from build123d import *

# Parameters (mm, degrees)
SKETCH1_R            = 36.5
BOSS_EXTRUDE1_DEPTH  = 5
SKETCH2_W            = 22
SKETCH2_H            = 14
CUT_EXTRUDE1_DEPTH   = 2.5
SKETCH6_W            = 14
SKETCH6_H            = 1.2
BOSS_EXTRUDE2_DEPTH  = 2.1
SKETCH7_W            = 14
SKETCH7_H            = 1.2
BOSS_EXTRUDE3_DEPTH  = 2.1
SKETCH8_W            = 14
SKETCH8_H            = 1.2
BOSS_EXTRUDE4_DEPTH  = 2.1
SKETCH10_W           = 14
SKETCH10_H           = 1.2
BOSS_EXTRUDE10_DEPTH = 2.1
SKETCH21_W           = 14
SKETCH21_H           = 1.2
BOSS_EXTRUDE11_DEPTH = 2.1
SKETCH13_W           = 14
SKETCH13_H           = 1.2
BOSS_EXTRUDE7_DEPTH  = 2.1
SKETCH14_W           = 14
SKETCH14_H           = 1.2
BOSS_EXTRUDE8_DEPTH  = 2.1
SKETCH18_W           = 14
SKETCH18_H           = 1.2
BOSS_EXTRUDE9_DEPTH  = 2.1
SKETCH20_R           = 36
CUT_EXTRUDE3_DEPTH   = 2.5
SKETCH22_R           = 1
CUT_EXTRUDE4_DEPTH   = 10
SKETCH24_R           = 1.7
CUT_EXTRUDE5_DEPTH   = 87.833561687


with BuildPart() as part:
    # Sketch1 → Boss-Extrude1 (new body)
    with BuildSketch(Plane(origin=(0, 0, 0), x_dir=(1, 0, 0), z_dir=(0, 1, 0))):
        with Locations(Location((33.33972472, -14.85640453, 0), (0, 0, 270))):
            Circle(SKETCH1_R)
    extrude(amount=BOSS_EXTRUDE1_DEPTH)

    # Sketch2 → Cut-Extrude1 (cut)
    with BuildSketch(Plane(origin=(0, 5, 0), x_dir=(1, 0, 0), z_dir=(0, 1, 0))):
        with Locations((36.135698514, -40.062546055)):
            Rectangle(SKETCH2_W, SKETCH2_H)
        with Locations((27.374405596, -24.326629568)):
            Rectangle(SKETCH2_W, SKETCH2_H)
        with Locations((27.467621635, 6.993959585)):
            Rectangle(SKETCH2_W, SKETCH2_H)
        with Locations((36.043497237, -8.573118952)):
            Rectangle(SKETCH2_W, SKETCH2_H)
    extrude(amount=-CUT_EXTRUDE1_DEPTH, mode=Mode.SUBTRACT)

    # Sketch6 → Boss-Extrude2 (add)
    with BuildSketch(Plane.ZY.offset(-38.467621635)):
        with Locations((-6.993959585, 4.4)):
            Rectangle(SKETCH6_W, SKETCH6_H)
    extrude(amount=BOSS_EXTRUDE2_DEPTH)

    # Sketch7 → Boss-Extrude3 (add)
    with BuildSketch(Plane(origin=(16.467621635, 0, 0), x_dir=(0, 0, -1), z_dir=(1, 0, 0))):
        with Locations((6.993959585, 4.4)):
            Rectangle(SKETCH7_W, SKETCH7_H)
    extrude(amount=BOSS_EXTRUDE3_DEPTH)

    # Sketch8 → Boss-Extrude4 (add)
    with BuildSketch(Plane(origin=(25.043497237, 0, 0), x_dir=(0, 0, -1), z_dir=(1, 0, 0))):
        with Locations((-8.573118952, 4.4)):
            Rectangle(SKETCH8_W, SKETCH8_H)
    extrude(amount=BOSS_EXTRUDE4_DEPTH)

    # Sketch10 → Boss-Extrude10 (add)
    with BuildSketch(Plane.ZY.offset(-47.043497237)):
        with Locations((8.573118952, 4.4)):
            Rectangle(SKETCH10_W, SKETCH10_H)
    extrude(amount=BOSS_EXTRUDE10_DEPTH)

    # Sketch21 → Boss-Extrude11 (add)
    with BuildSketch(Plane.ZY.offset(-38.374405596)):
        with Locations((24.326629568, 4.4)):
            Rectangle(SKETCH21_W, SKETCH21_H)
    extrude(amount=BOSS_EXTRUDE11_DEPTH)

    # Sketch13 → Boss-Extrude7 (add)
    with BuildSketch(Plane(origin=(16.374405596, 0, 0), x_dir=(0, 0, -1), z_dir=(1, 0, 0))):
        with Locations((-24.326629568, 4.4)):
            Rectangle(SKETCH13_W, SKETCH13_H)
    extrude(amount=BOSS_EXTRUDE7_DEPTH)

    # Sketch14 → Boss-Extrude8 (add)
    with BuildSketch(Plane.ZY.offset(-47.135698514)):
        with Locations((40.062546055, 4.4)):
            Rectangle(SKETCH14_W, SKETCH14_H)
    extrude(amount=BOSS_EXTRUDE8_DEPTH)

    # Sketch18 → Boss-Extrude9 (add)
    with BuildSketch(Plane(origin=(25.135698514, 0, 0), x_dir=(0, 0, -1), z_dir=(1, 0, 0))):
        with Locations((-40.062546055, 4.4)):
            Rectangle(SKETCH18_W, SKETCH18_H)
    extrude(amount=BOSS_EXTRUDE9_DEPTH)

    # Sketch20 → Cut-Extrude3 (cut)
    with BuildSketch(Plane.XZ):
        with Locations(Location((33.33972472, 14.85640453, 0), (0, 0, 270))):
            Circle(SKETCH20_R)
    extrude(amount=-CUT_EXTRUDE3_DEPTH, mode=Mode.SUBTRACT)

    # Sketch22 → Cut-Extrude4 (cut)
    with BuildSketch(Plane(origin=(0, 5, 0), x_dir=(1, 0, 0), z_dir=(0, 1, 0))):
        with Locations(Location((52.821638574, -38.573118952, 0), (0, 0, 270))):
            Circle(SKETCH22_R)
        with Locations(Location((10.967875326, -24.326629568, 0), (0, 0, 270))):
            Circle(SKETCH22_R)
        with Locations(Location((10.967875326, 5.673370432, 0), (0, 0, 270))):
            Circle(SKETCH22_R)
        with Locations(Location((52.821876902, -8.573118953, 0), (0, 0, 270))):
            Circle(SKETCH22_R)
    extrude(amount=-CUT_EXTRUDE4_DEPTH, mode=Mode.SUBTRACT)

    # Sketch24 → Cut-Extrude5 (cut, through all)
    with BuildSketch(Plane(origin=(0, 5, 0), x_dir=(1, 0, 0), z_dir=(0, 1, 0))):
        with Locations(Location((63.33972472, -14.85640453, 0), (0, 0, 270))):
            Circle(SKETCH24_R)
        with Locations(Location((3.33972472, -14.85640453, 0), (0, 0, 270))):
            Circle(SKETCH24_R)
    extrude(amount=-CUT_EXTRUDE5_DEPTH, mode=Mode.SUBTRACT)


solid = part.part
Can you work these out from the model? Positions are in its coordinate system, mm. A direction names the side the tool comes from. Give positions to 0.01 mm unless a question says otherwise; leave off trailing zeros. Loops run counter-clockwise (first coordinate to the right, second up) from the corner with the lowest first, then second, coordinate; pieces in that order, holes last. Notation, with made-up numbers: M -38,32 L 3,32 A28 cw 3,63 Z; hole C 49.5,44.25 d11. An arc over 180 degrees is marked long. One line per item, written item: value. Start each with the question number.
1) Thinking about a two-plate mould opening in X: for faces 1 (the face through (36, 4, 47.063)), 2 (the face through (44.3, 2.46, 49.67)), which applies, +X half, -X half, draft (parallel to the pull), parting line (faces both ways), or undercut?
2) If we section it at C-C, the plane x = 49: Write out the boundary of the cut face in (y, z).
3) If we section it at B-B, the plane x = 29: Write out the boundary of the cut face in (y, z), and give its area (3 significant figures).
4) If I drill on line 1 (X direction, y = 3.7, z = 9); line 2 (Z direction, x = 26, y = 3.3); line 3 (X direction, y = 3.25, z = 14), over which ranges is the centre line in solid material (lowest first)? Write a range as [from, to].
5) If we section it at D-D, the plane z = 22: Write out the boundary of the cut face in (x, y), and give its area (3 significant figures).
6) I'm going to push flat-ended pins straight in: pin 1 (1 mm diameter, centred on y = 3.5, z = 24.5, fed in from +X); pin 2 (2 mm diameter, centred on x = 3.34, z = 14.86, fed in from -Y); pin 3 (1 mm diameter, centred on y = 4.5, z = 25.5, fed in from -X); pin 4 (1.2 mm diameter, centred on x = 31, y = 4, fed in from +Z). Where does each tip first touch, or does it pass through?
7) If we section it at A-A, the plane z = -9: Write out the boundary of the cut face in (x, y), and give its area (3 significant figures).
8) On a 3-axis mill with a long thin cutter (end or side, diameter ignored), from which of +Z, -Z, +X, -X, +Y, -Y can I reach the whole of each face in a straight line? I mean faces 3 (the face through (52, 4, 38)), 4 (the face through (36, 4, 1.573)). Say none if no direction works.
Completed:
1. face 1: undercut
1. face 2: parting line
2. outline: M 0,-18.11 L 5,-18.11 L 5,47.83 L 0,47.83 L 0,47.27 L 2.5,47.27 L 2.5,-17.56 L 0,-17.56 Z
3. outline: M 0,-21.38 L 5,-21.38 L 5,-13.99 L 2.5,-13.99 L 2.5,-20.88 L 0,-20.88 Z; M 0,50.59 L 2.5,50.59 L 2.5,47.06 L 5,47.06 L 5,51.1 L 0,51.1 Z; M 2.5,0.01 L 5,0.01 L 5,1.57 L 2.5,1.57 Z; M 2.5,15.57 L 5,15.57 L 5,17.33 L 2.5,17.33 Z; M 2.5,31.33 L 5,31.33 L 5,33.06 L 2.5,33.06 Z
3. area: 43.7 mm^2
4. line 1: x = [-2.69, 25.04], [47.04, 51.92], [53.73, 69.37]
4. line 2: z = [-20.9, -13.99], [0.01, 1.57], [15.57, 17.33], [31.33, 33.06], [47.06, 50.61]
4. line 3: x = [-3.15, 1.87], [4.81, 25.04], [47.04, 61.87], [64.81, 69.83]
5. outline: M -2.45,0 L -1.94,0 L -1.94,2.5 L 16.37,2.5 L 16.37,3.8 L 18.47,3.8 L 18.47,5 L -2.45,5 Z; M 36.27,3.8 L 38.37,3.8 L 38.37,2.5 L 68.62,2.5 L 68.62,0 L 69.13,0 L 69.13,5 L 36.27,5 Z
5. area: 132 mm^2
6. pin 1: stops at x = 68.68
6. pin 2: passes through
6. pin 3: stops at x = -1.72
6. pin 4: stops at z = 51.31
7. outline: M 5.72,0 L 6.38,0 L 6.38,2.5 L 16.47,2.5 L 16.47,3.8 L 18.57,3.8 L 18.57,5 L 5.72,5 Z; M 36.37,3.8 L 38.47,3.8 L 38.47,2.5 L 60.3,2.5 L 60.3,0 L 60.96,0 L 60.96,5 L 36.37,5 Z
7. area: 91.5 mm^2
8. face 3: +Y, -Y
8. face 4: -Y
